Geometry check sheet. Reference: the model listing, model coordinates, mm. A direction names the side the tool comes from. Round coordinates to 2 decimals unless told otherwise and drop trailing zeros. Order: outer loops, then holes, each group sorted by start corner. A loop starts at its lowest first (then second) coordinate and runs counter-clockwise, first axis right, second up. Notation, with made-up numbers: (-23, -36) - (-10, -36) arc R15 ccw to (-10, -24) - close; hole circle Ø9 at (-8.75, -3.75). An arc over 180 degrees is marked (long way). Return JSON: item names as keys, results as strings. Group by question number.
Q1. Sectioned sample at B-B, the plane z = 432. Record the cut outline in (x, y).
Q2. Sectioned sample at C-C, the plane z = 307.5. Record the cut outline in (x, y).
Q3. Sectioned sample at D-D, the plane z = 88. Record the cut outline in (x, y), then the cut area to 3 significant figures.
Q4. Material ranges on line 1 along Z through (x, y) = (-363, 594); line 2 along Y through (x, z) = (24, 263.5); line 3 along X through (y, z) = (317, 202), recorded low to high.
Q5. Sectioned sample at A-A, the plane x = 0. Record the cut outline in (y, z).
Q6. Tool access check on faces 4 (the flat face through (-367.555, 435.952, 424.966)), 5 (the flat face through (438.062, 365.037, 424.966)), 6 (the flat face through (349.47, 293.76, 181.77)), 7 (the flat face through (-148, 533, 560)), 8 (the flat face through (-438.062, -365.037, 424.966)). Record the directions out of +Z, -Z, +X, -X, +Y, -Y that give a thin tool (end or side, any length) a straight path to the whole face; none if there is none.
Q7. Gauge pin test, flat ends, axial feed: pin 1 Ø8 at (y, z) = (-73.5, 533) entering from +X; pin 2 Ø5.5 at (x, y) = (-219.5, 4.5) entering from -Z; pin 3 Ø6 at (x, z) = (-262.5, 529.5) entering from +Y. Record the tip position at first contact, or that the pin passes through.
Q8. Draft check along X on faces 1 (the flat face through (-418.105, 416.69, 372.043)), 2 (the flat face through (419.092, -415.697, 372.043)), 3 (the cylindrical face through (-588.26, -567.75, 609.3)). Enter one of: pulls with the +X half, pulls with the -X half, needs draft (parallel to the pull), parting line crosses it, or undercut.
```python
from build123d import *

# Parameters (mm, degrees)
SCHIZZO1_R                      = 400
ESTRUSIONE_ESTRUSIONE2_DEPTH    = 10
SCHIZZO2_R                      = 550
ESTRUSIONE_ESTRUSIONE3_DEPTH    = 550
ESTRUSIONE_ESTRUSIONE3_DRAFT    = -14
SCHIZZO7_W                      = 1307.512156596
SCHIZZO7_H                      = 1300
SCHIZZO7_R                      = 550
ESTRUSIONE_ESTRUSIONE4_DEPTH    = 100
ESTRUSIONE_ESTRUSIONE15_DEPTH   = 50
SCHIZZO16_R                     = 40
TAGLIO_ESTRUSIONE1_DEPTH        = 183
ESTRUSIONE_ESTRUSIONE21_DEPTH   = 50
ESTRUSIONE_ESTRUSIONE23_DEPTH   = 50
ESTRUSIONE_ESTRUSIONE23_2_DEPTH = 50
RIPETIZIONECIRCOLARE3_COUNT     = 4
SCHIZZO19_R                     = 550
ESTRUSIONE_ESTRUSIONE24_DEPTH   = 100
RACCORDO1_R                     = 13


with BuildPart() as part:
    # Schizzo1 → Estrusione-Estrusione2 (new body)
    with BuildSketch(Plane.XY.offset(10)):
        Circle(SCHIZZO1_R)
        with BuildLine():
            ThreePointArc((159.461880199, 183.128480143), (168.874067872, 192.540667817), (159.461880199, 201.952855491))
            ThreePointArc((159.461880199, 201.952855491), (150.049692525, 192.540667817), (159.461880199, 183.128480143))
        make_face(mode=Mode.SUBTRACT)
        with BuildLine():
            ThreePointArc((142.354854673, 173.854716695), (132.942666999, 164.442529021), (142.354854673, 155.030341347))
            ThreePointArc((142.354854673, 155.030341347), (151.767042347, 164.442529021), (142.354854673, 173.854716695))
        make_face(mode=Mode.SUBTRACT)
        with BuildLine():
            ThreePointArc((142.354854673, -155.030341347), (132.942666999, -164.442529021), (142.354854673, -173.854716695))
            ThreePointArc((142.354854673, -173.854716695), (151.767042347, -164.442529021), (142.354854673, -155.030341347))
        make_face(mode=Mode.SUBTRACT)
        with BuildLine():
            ThreePointArc((159.461880199, -183.128480143), (150.049692525, -192.540667817), (159.461880199, -201.952855491))
            ThreePointArc((159.461880199, -201.952855491), (168.874067872, -192.540667817), (159.461880199, -183.128480143))
        make_face(mode=Mode.SUBTRACT)
        with BuildLine():
            ThreePointArc((-217.5, 9.412187674), (-226.912187674, 0), (-217.5, -9.412187674))
            ThreePointArc((-217.5, -9.412187674), (-208.087812326, 0), (-217.5, 9.412187674))
        make_face(mode=Mode.SUBTRACT)
        with BuildLine():
            ThreePointArc((-250, 9.412187674), (-259.412187674, 0), (-250, -9.412187674))
            ThreePointArc((-250, -9.412187674), (-240.587812326, 0), (-250, 9.412187674))
        make_face(mode=Mode.SUBTRACT)
    extrude(amount=-ESTRUSIONE_ESTRUSIONE2_DEPTH)


with BuildPart() as estrusione_estrusione3_tool:
    # Schizzo2 → Estrusione-Estrusione3 (with draft: the straight prism first)
    with BuildSketch(Plane.XY.offset(560)):
        Circle(SCHIZZO2_R)
    extrude(amount=-ESTRUSIONE_ESTRUSIONE3_DEPTH)
    # Estrusione-Estrusione3: the draft: its side faces are tilted about the plane it starts from
    estrusione_estrusione3_sides = [estrusione_estrusione3_tool.faces().sort_by_distance(p)[0] for p in [
        (-550, 0, 285),
    ]]
    draft(estrusione_estrusione3_sides, Plane.XY.offset(560), ESTRUSIONE_ESTRUSIONE3_DRAFT)


with BuildPart() as part_1:
    add(part.part)

    # Estrusione-Estrusione3: add estrusione_estrusione3_tool
    add(estrusione_estrusione3_tool.part)



with BuildPart() as body_2:
    # Schizzo7 → Estrusione-Estrusione4 (new body)
    with BuildSketch(Plane.XY.offset(560)):
        Rectangle(SCHIZZO7_W, SCHIZZO7_H)
        Circle(SCHIZZO7_R, mode=Mode.SUBTRACT)
    extrude(amount=ESTRUSIONE_ESTRUSIONE4_DEPTH)

    # Schizzo16 → Taglio-Estrusione1 (cut)
    with BuildSketch(Plane(origin=(0, 0, 560), x_dir=(-1, 0, 0), z_dir=(0, 0, -1))):
        with Locations((-606.722155674, 603.236305221)):
            Circle(SCHIZZO16_R)
    taglio_estrusione1 = extrude(amount=-TAGLIO_ESTRUSIONE1_DEPTH, mode=Mode.SUBTRACT)

    # RipetizioneCircolare3: Taglio-Estrusione1 ×4 about axis
    ripetizionecircolare3_axis = Axis((0, 0, 0), (0, 0, 1))
    for i in range(1, RIPETIZIONECIRCOLARE3_COUNT):
        add(taglio_estrusione1.rotate(ripetizionecircolare3_axis, i * 360 / RIPETIZIONECIRCOLARE3_COUNT), mode=Mode.SUBTRACT)


with BuildPart() as body_3:
    # Schizzo15 → Estrusione-Estrusione15 (new, symmetric)
    with BuildSketch(Plane(origin=(0, 0, 0), x_dir=(-0.7091409896026719, -0.7050667038410928, 0), z_dir=(0.7050667038410928, -0.7091409896026719, 0))):
        Polygon((-721.89858982, -560), (-454.943274801, -178.748298966), (-454.943274801, -560), align=None)
    extrude(amount=ESTRUSIONE_ESTRUSIONE15_DEPTH, both=True)


with BuildPart() as body_4:
    # Schizzo17 → Estrusione-Estrusione21 (new, symmetric)
    with BuildSketch(Plane(origin=(0, 0, 0), x_dir=(-0.7091409896026719, -0.7050667038410928, 0), z_dir=(0.7050667038410928, -0.7091409896026719, 0))):
        Polygon((721.89858982, -560), (454.943274801, -178.748298966), (454.943274801, -560), align=None)
    extrude(amount=ESTRUSIONE_ESTRUSIONE21_DEPTH, both=True)


with BuildPart() as body_5:
    # Schizzo18 → Estrusione-Estrusione23 (new, symmetric)
    with BuildSketch(Plane(origin=(0, 0, 0), x_dir=(0.7091409896026718, -0.7050667038410929, 0), z_dir=(0.7050667038410929, 0.7091409896026718, 0))):
        Polygon((-721.89858982, -560), (-454.943274801, -178.748298966), (-454.943274801, -560), align=None)
    extrude(amount=ESTRUSIONE_ESTRUSIONE23_DEPTH, both=True)


with BuildPart() as body_6:
    # Schizzo18 → Estrusione-Estrusione23 2 (new, symmetric)
    with BuildSketch(Plane(origin=(0, 0, 0), x_dir=(0.7091409896026718, -0.7050667038410929, 0), z_dir=(0.7050667038410929, 0.7091409896026718, 0))):
        Polygon((721.89858982, -560), (454.943274801, -178.748298966), (454.943274801, -560), align=None)
    extrude(amount=ESTRUSIONE_ESTRUSIONE23_2_DEPTH, both=True)


with BuildPart() as part_2:
    add(part_1.part)

    add(body_2.part)  # Estrusione-Estrusione24 merges body 2

    add(body_3.part)  # Estrusione-Estrusione24 merges body 3

    add(body_4.part)  # Estrusione-Estrusione24 merges body 4

    add(body_5.part)  # Estrusione-Estrusione24 merges body 5

    add(body_6.part)  # Estrusione-Estrusione24 merges body 6
    # Schizzo19 → Estrusione-Estrusione24 (add)
    with BuildSketch(Plane.XY.offset(560)):
        Circle(SCHIZZO19_R)
    extrude(amount=ESTRUSIONE_ESTRUSIONE24_DEPTH)

    # Raccordo1
    # the kernel refuses this fillet: 13 mm, written as the material it adds along each edge
    with BuildSketch(Plane(origin=(0, 0, 10), x_dir=(1, 0, 0), z_dir=(0, -1, 0))) as raccordo1_piece_1:
        with BuildLine():
            CenterArc((412.649110641, -13), RACCORDO1_R, 90, 76.657636203)
            Line((400, -10), (400, 0))
            Line((400, 0), (412.649110641, 0))
        make_face()
    revolve(axis=Axis((0, 0, 10), (0, 0, 1)))


solid = part_2.part
```
Reply:
{
 "1": {"outline": "(-483.62, -410.34) - (-413.12, -481.25) - (-330.43, -399.04) arc R518.09 ccw to (330.43, -399.04) - (413.12, -481.25) - (483.62, -410.34) - (400.93, -328.12) arc R518.09 ccw to (400.93, 328.12) - (483.62, 410.34) - (413.12, 481.25) - (330.43, 399.04) arc R518.09 ccw to (-330.43, 399.04) - (-413.12, 481.25) - (-483.62, 410.34) - (-400.93, 328.12) arc R518.09 ccw to (-400.93, -328.12) - close"},
 "2": {"outline": "(-421.8, -348.87) - (-351.3, -419.79) - (-308.31, -377.04) arc R487.04 ccw to (308.31, -377.04) - (351.3, -419.79) - (421.8, -348.87) - (378.81, -306.13) arc R487.04 ccw to (378.81, 306.13) - (421.8, 348.87) - (351.3, 419.79) - (308.31, 377.04) arc R487.04 ccw to (-308.31, 377.04) - (-351.3, 419.79) - (-421.8, 348.87) - (-378.81, 306.13) arc R487.04 ccw to (-378.81, -306.13) - close"},
 "3": {"outline": "circle Ø864.63 at (0, 0)", "area": "587,000 mm^2"},
 "4": {"line 1": "560 to 660", "line 2": "-475.47 to 475.47", "line 3": "-349.32 to 349.32"},
 "5": {"outline": "(-650, 560) - (-550, 560) - (-412.87, 10) - (-412.65, 10) arc R13 cw to (-400, 0) - (400, 0) arc R13 cw to (412.65, 10) - (412.87, 10) - (550, 560) - (650, 560) - (650, 660) - (-650, 660) - close"},
 "6": {"face 4": "-Z, +Y", "face 5": "-Z, +X", "face 6": "none", "face 7": "-Z", "face 8": "-Z, -X"},
 "7": {"pin 1": "x = 539.41", "pin 2": "z = 10", "pin 3": "y = 476.5"},
 "8": {"face 1": "pulls with the -X half", "face 2": "pulls with the +X half", "face 3": "undercut"}
}
